```python
from build123d import *

# Parameters (mm, degrees)
F1_DEPTH = 100
F2_R     = 6
F3_DEPTH = 25


with BuildPart() as f1:
    # F0 (on Right) → F1 (new body)
    with BuildSketch(Plane.YZ):
        Polygon((9, 0), (0, 0), (0, -38.9847982002), (120, -38.9847982002), (120, -29.9847982002), (9, -29.9847982002), align=None)
    extrude(amount=F1_DEPTH)

    # F2 (on face) → F3 (cut)
    with BuildSketch(Plane.XZ):
        with Locations((20, -19.4923991001)):
            Circle(F2_R)
        with Locations((80, -19.4923991001)):
            Circle(F2_R)
    extrude(amount=-F3_DEPTH, mode=Mode.SUBTRACT)


solid = f1.part
```
Source: CAD feature listing. Evaluate the final solid. Frame: model axes, mm. A direction names the side the tool comes from. Give positions to 0.01 mm unless a question says otherwise; leave off trailing zeros. Write each loop counter-clockwise with the first axis right and the second up, starting at its lowest first coordinate (ties: lowest second). Pieces come first, ordered by that corner, then holes. Notation, with made-up numbers: (-11, -1.5) - (14, -1.5) arc R5 cw to (14, 5.5) - close; hole circle Ø5 at (64.25, -39). An arc over 180 degrees is marked (long way). One line per item, written item: value. Start each with the question number.
Q1. Material intervals for probe 1 along Z at (x, y) = (20, 7.25); probe 2 along Z at (x, y) = (16.5, 12.5); probe 3 along Y at (x, z) = (35.5, -4), sorted ascending. Write a range as from..to.
Q2. Section query D-D, the plane x = 36. Return the cut outline in (y, z).
Q3. First-contact query: pin 1 Ø5 at (x, z) = (56, -17.5) entering from +Y; pin 2 Ø4 at (x, y) = (25, 17.5) entering from +Z. Flat tips, straight axial feed; report the tip coordinate or a pass-through.
Q4. Draft query along Z for faces 3 (the face through (49, 9, -15)), 4 (the face through (22.8, 4.4, -24.8)), 5 (the face through (74.006, 4.437, -19.229)), 6 (the face through (49, 5, 0)). Return one class per face: +Z half, -Z half, draft (parallel to the pull), parting line (faces both ways), or undercut.
Q5. Section query B-B, the plane z = -6. Return the cut outline in (x, y).
Q6. Set-up query: faces 1 (the face through (49, 65, -29.985)), 2 (the face through (100, 46, -31)). Return all of +Z, -Z, +X, -X, +Y, -Y with unobstructed straight access to the full face (end or side cutting, diameter ignored); none if empty.
Q7. Section query C-C, the plane y = 38.5. Return the cut outline in (x, z), then the cut area to 3 significant figures.
Q8. Section query A-A, the plane x = 20. Return the cut outline in (y, z).
Answer:
1. probe 1: z = -38.98..-25.49, -13.49..0
1. probe 2: z = -38.98..-29.98
1. probe 3: y = 0..9
2. outline: (0, -38.98) - (120, -38.98) - (120, -29.98) - (9, -29.98) - (9, 0) - (0, 0) - close
3. pin 1: stops at y = 9
3. pin 2: stops at z = -29.98
4. face 3: draft
4. face 4: undercut
4. face 5: undercut
4. face 6: +Z half
5. outline: (0, 0) - (100, 0) - (100, 9) - (0, 9) - close
6. face 1: +Z, +X, -X, +Y
6. face 2: +Z, -Z, +X, +Y, -Y
7. outline: (0, -38.98) - (100, -38.98) - (100, -29.98) - (0, -29.98) - close
7. area: 900 mm2
8. outline: (0, -38.98) - (120, -38.98) - (120, -29.98) - (9, -29.98) - (9, -25.49) - (0, -25.49) - close; (0, -13.49) - (9, -13.49) - (9, 0) - (0, 0) - close
